```python
from build123d import *

# Parameters (mm, degrees)
SKETCH1_R           = 1.5
BOSS_EXTRUDE1_DEPTH = 2
CUT_EXTRUDE1_DEPTH  = 2
BOSS_EXTRUDE2_REACH = 13.18
SKETCH3_W           = 14
SKETCH3_H           = 1
FILLET1_SIZE        = 1


with BuildPart() as part:
    # Sketch1 → Boss-Extrude1 (new, symmetric)
    with BuildSketch(Plane(origin=(0, 0, 0), x_dir=(1, 0, 0), z_dir=(0, 1, 0))):
        with BuildLine():
            Line((-7, 3), (7, 3))
            ThreePointArc((7, 3), (10, 0), (7, -3))
            Line((7, -3), (-7, -3))
            ThreePointArc((-7, -3), (-10, 0), (-7, 3))
        make_face()
        with Locations(Location((-7, 0, 0), (0, 0, 270))):
            Circle(SKETCH1_R, mode=Mode.SUBTRACT)
        with Locations(Location((7, 0, 0), (0, 0, 270))):
            Circle(SKETCH1_R, mode=Mode.SUBTRACT)
    extrude(amount=BOSS_EXTRUDE1_DEPTH, both=True)

    # Sketch2 → Cut-Extrude1 (cut)
    with BuildSketch(Plane(origin=(0, 2, 0), x_dir=(1, 0, 0), z_dir=(0, 1, 0))):
        with BuildLine():
            Line((5.197224362, 3), (7, 3))
            ThreePointArc((7, 3), (10, 0), (7, -3))
            Line((7, -3), (5.197224362, -3))
            ThreePointArc((5.197224362, -3), (3.5, 0), (5.197224362, 3))
        make_face()
    extrude(amount=-CUT_EXTRUDE1_DEPTH, mode=Mode.SUBTRACT)

    # Boss-Extrude2: up to this face of the body (flat: up to its plane)
    boss_extrude2_end = Plane(part.part.faces().sort_by_distance((-2.270949872, 2, 0))[0])
    # Sketch3 → Boss-Extrude2 (add, up to the picked face)
    with BuildSketch(Plane.XZ.offset(2), mode=Mode.PRIVATE) as boss_extrude2_sk1:
        with Locations((0, -3.5)):
            Rectangle(SKETCH3_W, SKETCH3_H)
    boss_extrude2_tool1 = split(extrude(boss_extrude2_sk1.sketch, amount=-BOSS_EXTRUDE2_REACH, mode=Mode.PRIVATE), bisect_by=boss_extrude2_end, keep=Keep.BOTH, mode=Mode.PRIVATE)
    add(boss_extrude2_tool1.solids().sort_by(Axis((0, -2, -3.5), (0, 1, 0)))[0])

    # Fillet1
    # a fillet whose section is not a circle: 1 mm, written as the material it takes off along each edge
    with BuildSketch(Plane(origin=(7, -4.5, -4), x_dir=(0, 0, 1), z_dir=(0, 1, 0)), Plane(origin=(-7, -4.5, -4), x_dir=(1, 0, 0), z_dir=(0, 1, 0))) as fillet1_piece_1:
        with BuildLine():
            add(Edge.make_bspline([(FILLET1_SIZE, 0), (FILLET1_SIZE * 0.831801948466, 0), (FILLET1_SIZE * 0.663603896932, 0), (FILLET1_SIZE * 0.292893218813, -FILLET1_SIZE * 0.0716919198361), (FILLET1_SIZE * 0.0716919198361, -FILLET1_SIZE * 0.292893218813), (0, -FILLET1_SIZE * 0.663603896932), (0, -FILLET1_SIZE * 0.831801948466), (0, -FILLET1_SIZE)], knots=[0, 0, 0, 0, 0, 0, 0.5, 0.5, 1, 1, 1, 1, 1, 1], degree=5))
            Line((0, -FILLET1_SIZE), (0, 0))
            Line((0, 0), (FILLET1_SIZE, 0))
        make_face()
    extrude(amount=9, mode=Mode.SUBTRACT)


solid = part.part
```
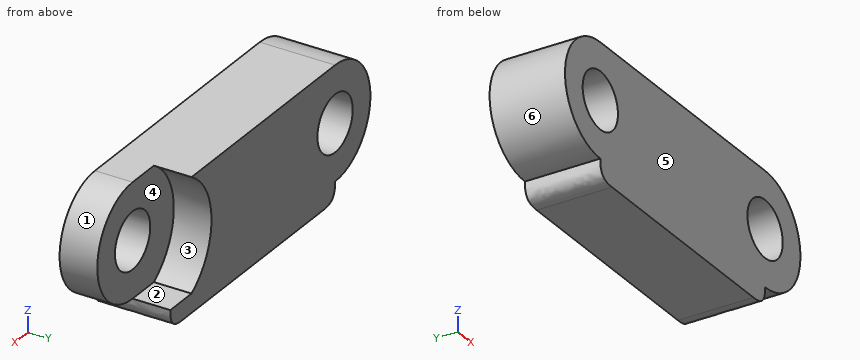
CAD build for the part. Positions are in the model's coordinates, mm. Face numbers are marked on the shaded views. A direction names the side the tool comes from. Round coordinates to 2 decimals unless told otherwise and drop trailing zeros. Loops run counter-clockwise (first coordinate to the right, second up) from the corner with the lowest first, then second, coordinate; pieces in that order, holes last. Notation, with made-up numbers: (30, 26.5) - (61, 26.5) arc R8 cw to (61, 34.5) - close; hole circle Ø5 at (14.5, 54.5). An arc over 180 degrees is marked (long way). Return JSON: item names as keys, results as strings. Group by question number.
Q1. Band-saw the part on D-D on y = -0.7. Give the number of separate pieces and of enclosed holes in the cut face, plus the area to 3 significant figures.
Q2. Band-saw the part on A-A on x = -8.25. Give the cut face in (y, z), plus the area to 3 significant figures.
Q3. Tool access for the marked faces 1, 2 and 3: list every direction of +Z, -Z, +X, -X, +Y, -Y with a clear straight run to the whole face (end or side of a thin tool).
Q4. Band-saw the part on C-C on x = 4.75. Give the cut face in (y, z).
Q5. Flat gauge pins, fed straight in: pin 1 Ø2 at (x, z) = (7, 1) entering from +Y; pin 2 Ø2 at (y, z) = (1.5, -2.5) entering from -X. Where does each tip first touch, or does it go through?
Q6. Drill centre lines: line 1 along X through (y, z) = (-0.95, 0); line 2 along X through (y, z) = (-0.5, 1.25); line 3 along X through (y, z) = (1.7, 0). Where is each one in solid material? Low to high. Write a range as [from, to].
Q7. Band-saw the part on B-B on z = 1.25. Give the cut face in (x, y).
Q8. Two-plate mould, pull along Z, no slides. Class the marked faces 4, 5 and 6: +Z half, -Z half, draft (parallel to the pull), parting line (faces both ways), or undercut.
Solutions:
{
 "1": {"separate pieces": "1", "enclosed holes": "2", "area": "112 mm^2"},
 "2": {"outline": "(-2, -2.73) - (2, -2.73) - (2, -0.83) - (-2, -0.83) - close; (-2, 0.83) - (2, 0.83) - (2, 2.73) - (-2, 2.73) - close", "area": "15.2 mm^2"},
 "3": {"face 1": "+X, +Y, -Y", "face 2": "+Z, +X, +Y", "face 3": "+X, +Y"},
 "4": {"outline": "(-2, -4) - (2, -4) - (2, -2.68) - (0, -2.68) - (0, 2.68) - (2, 2.68) - (2, 3) - (-2, 3) - close"},
 "5": {"pin 1": "stops at y = 0", "pin 2": "stops at x = -9.6"},
 "6": {"line 1": "x = [-10, -8.5], [-5.5, 5.5], [8.5, 10]", "line 2": "x = [-9.73, -7.83], [-6.17, 6.17], [7.83, 9.73]", "line 3": "x = [-10, -8.5], [-5.5, 3.5]"},
 "7": {"outline": "(-9.73, -2) - (-7.83, -2) - (-7.83, 2) - (-9.73, 2) - close; (-6.17, -2) - (6.17, -2) - (6.17, 0) - (3.73, 0) - (3.73, 2) - (-6.17, 2) - close; (7.83, -2) - (9.73, -2) - (9.73, 0) - (7.83, 0) - close"},
 "8": {"face 4": "undercut", "face 5": "draft", "face 6": "parting line"}
}
